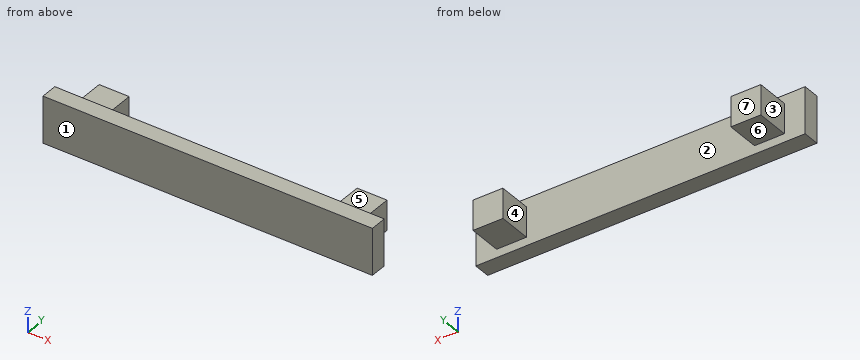
```python
from build123d import *

# Parameters (mm, degrees)
SKETCH1_W           = 19.8
SKETCH1_H           = 2.8
SKETCH1_W_2         = 1.8
SKETCH1_H_2         = 1.8
BOSS_EXTRUDE1_DEPTH = 1
SKETCH1_3_W         = 1.8
SKETCH1_3_H         = 1.8
BOSS_EXTRUDE2_DEPTH = 3


with BuildPart() as part:
    # Sketch1 → Boss-Extrude1 (new body)
    with BuildSketch(Plane(origin=(0, 0, 0), x_dir=(1, 0, 0), z_dir=(0, 1, 0))):
        with Locations((9.9, 1.4)):
            Rectangle(SKETCH1_W, SKETCH1_H)
        with Locations((2.15, 1.4)):
            Rectangle(SKETCH1_W_2, SKETCH1_H_2, mode=Mode.SUBTRACT)
        with Locations((17.65, 1.4)):
            Rectangle(SKETCH1_W_2, SKETCH1_H_2, mode=Mode.SUBTRACT)
    extrude(amount=BOSS_EXTRUDE1_DEPTH)

    # Sketch1<3> → Boss-Extrude2 (add)
    with BuildSketch(Plane(origin=(0, 0, 0), x_dir=(1, 0, 0), z_dir=(0, 1, 0))):
        with Locations((2.15, 1.4)):
            Rectangle(SKETCH1_3_W, SKETCH1_3_H)
        with Locations((17.65, 1.4)):
            Rectangle(SKETCH1_3_W, SKETCH1_3_H)
    extrude(amount=BOSS_EXTRUDE2_DEPTH)


solid = part.part
```
Design review of the part built by this model. Coordinates are the model's own, in mm. Face numbers are marked on the shaded views. A direction names the side the tool comes from. Give positions to 0.01 mm unless a question says otherwise; leave off trailing zeros. Loops run counter-clockwise (first coordinate to the right, second up) from the corner with the lowest first, then second, coordinate; pieces in that order, holes last. Notation, with made-up numbers: M 0.5,9.5 L 58.5,9.5 A16 cw 58.5,28.5 Z; hole C -28.75,8.25 d1. An arc over 180 degrees is marked long. Return JSON: item names as keys, results as strings. Group by question number.
Item 1: We need section A-A (y = 2.1). Give the boundary of the cut face in (x, z).
Item 2: Mouldability with a two-part tool opening along X and no side actions: class the marked faces 1, 2, 3 and 4 as released by +X, released by -X, zero draft, split by the parting line, or undercut.
Item 3: For probe 1 along X at (y, z) = (1.4, -1.25); probe 2 along Y at (x, z) = (9, -1.85); probe 3 along Z at (x, y) = (1.5, 1.5), list the stretches that pass through material, from the lowest coordinate up.
Item 4: We need section B-B (x = 1.75). Give the boundary of the cut face in (y, z), and give its area (3 significant figures).
Item 5: Tool access review of the marked faces 5, 6 and 7: name each direction out of +Z, -Z, +X, -X, +Y, -Y from which nothing blocks a thin tool from reaching the whole face with its end or side.
Item 6: We need section D-D (z = -2.5). Give the boundary of the cut face in (x, y).
Item 7: Insertion check: pin 1 Ø0.5 at (x, y) = (2.5, 1.5) entering from +Z; pin 2 Ø0.5 at (x, y) = (18, 2) entering from -Z; pin 3 Ø0.9 at (y, z) = (2, -2) entering from -X. Each pin has a flat end and moves straight along its axis. Give the tip position at first contact, or say it passes through.
Item 8: We need section C-C (z = -1.15). Give the boundary of the cut face in (x, y), and give its area (3 significant figures).
Output:
{
 "1": {"outline": "M 1.25,-2.3 L 3.05,-2.3 L 3.05,-0.5 L 1.25,-0.5 Z; M 16.75,-2.3 L 18.55,-2.3 L 18.55,-0.5 L 16.75,-0.5 Z"},
 "2": {"face 1": "zero draft", "face 2": "undercut", "face 3": "released by -X", "face 4": "undercut"},
 "3": {"probe 1": "x = 1.25 to 3.05, 16.75 to 18.55", "probe 2": "y = 0 to 1", "probe 3": "z = -2.3 to -0.5"},
 "4": {"outline": "M 0,-2.8 L 1,-2.8 L 1,-2.3 L 3,-2.3 L 3,-0.5 L 1,-0.5 L 1,0 L 0,0 Z", "area": "6.40 mm^2"},
 "5": {"face 5": "+Z, +X, -X, +Y", "face 6": "-Z, +X, -X, +Y", "face 7": "+Z, -Z, +X, -X, +Y"},
 "6": {"outline": "M 0,0 L 19.8,0 L 19.8,1 L 0,1 Z"},
 "7": {"pin 1": "stops at z = -0.5", "pin 2": "stops at z = -2.3", "pin 3": "stops at x = 1.25"},
 "8": {"outline": "M 0,0 L 19.8,0 L 19.8,1 L 18.55,1 L 18.55,3 L 16.75,3 L 16.75,1 L 3.05,1 L 3.05,3 L 1.25,3 L 1.25,1 L 0,1 Z", "area": "27.0 mm^2"}
}
